The model under review builds one solid part; all positions refer to its coordinate system, in mm. Coordinates: 2 decimals unless noted, no trailing zeros. Loops run counter-clockwise (first coordinate to the right, second up) from the corner with the lowest first, then second, coordinate; pieces in that order, holes last. Notation, with made-up numbers: (-30.75, 23.5) - (26.25, 23.5) arc R18 ccw to (26.25, 42.5) - close; hole circle Ø5 at (58, 81.25). An arc over 180 degrees is marked (long way). Use a Markdown table: item, result. Add a question column.
1) Add section A-A, the plane z = -15.5. Give the boundary of the cut face in (x, y), and give its area (3 significant figures).
2) Clearance check with flat-ended pins moving along their axes: pin 1 (1 mm diameter, centred on x = -0.5, y = 0.5, fed in from -Z); pin 2 (2 mm diameter, centred on x = 0, y = 0, fed in from -Z); pin 3 (1 mm diameter, centred on x = -2, z = 10, fed in from -Y). State where each tip first meets the part, or that it passes through.
3) Add section C-C, the plane y = -1.95. Give the boundary of the cut face in (x, z), and give its area (3 significant figures).
4) Add section D-D, the plane x = 1.7. Give the boundary of the cut face in (y, z).
5) To check wall thickness, follow L1, parallel to Y at x = 0, z = -17; L2, parallel to Y at x = 0.5, z = -14; L3, parallel to Y at x = 1.6, z = -15. State the ranges of each line that lie inside material, in increasing order. Write a range as [from, to].
6) Add section B-B, the plane z = 6. Give the boundary of the cut face in (x, y).
```python
from build123d import *

# Parameters (mm, degrees)
SKETCH_6_R               = 2.5
EXTRUDE_2_DEPTH          = 19.3
M3X0_5_3_D               = 2.5
M3X0_5_3_DEPTH           = 8.5
M3X0_5_3_TIP             = 0.751075774
M3X0_5_3_ON_FACE_2_D     = 2.5
M3X0_5_3_ON_FACE_2_DEPTH = 8.5
M3X0_5_3_ON_FACE_2_TIP   = 0.751075774


with BuildPart() as part:
    # ｽｹｯﾁ6 → ﾎﾞｽ - 押し出し2 (new body, symmetric)
    with BuildSketch(Plane.XY):
        Circle(SKETCH_6_R)
    extrude(amount=EXTRUDE_2_DEPTH, both=True)

    # M3x0.5 ねじ穴3
    with Locations(Plane.XY.offset(19.3)):
        with Locations((0, 0)):
            Hole(M3X0_5_3_D / 2, depth=M3X0_5_3_DEPTH)
            with Locations((0, 0, -(M3X0_5_3_DEPTH + M3X0_5_3_TIP / 2))):  # 118° drill point
                Cone(0, M3X0_5_3_D / 2, M3X0_5_3_TIP, mode=Mode.SUBTRACT)

    # M3x0.5 ねじ穴3 on face 2
    with Locations(Plane(origin=(0, 0, -19.3), x_dir=(-1, 0, 0), z_dir=(0, 0, -1))):
        with Locations((0, 0)):
            Hole(M3X0_5_3_ON_FACE_2_D / 2, depth=M3X0_5_3_ON_FACE_2_DEPTH)
            with Locations((0, 0, -(M3X0_5_3_ON_FACE_2_DEPTH + M3X0_5_3_ON_FACE_2_TIP / 2))):  # 118° drill point
                Cone(0, M3X0_5_3_ON_FACE_2_D / 2, M3X0_5_3_ON_FACE_2_TIP, mode=Mode.SUBTRACT)


solid = part.part
```
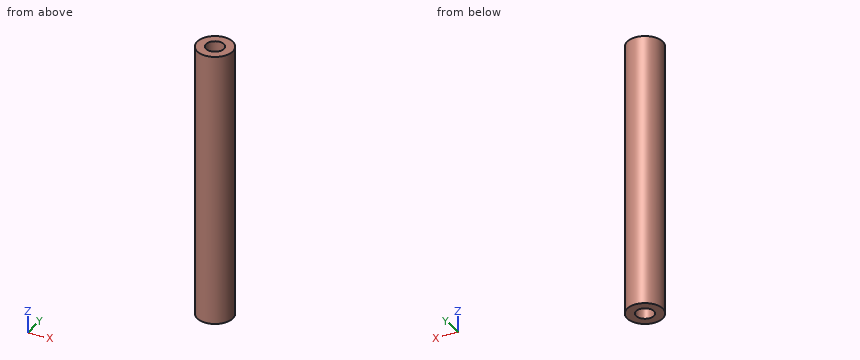
From the geometry:
| question | item | result |
|---|---|---|
| 1 | outline | circle Ø5 at (0, 0); hole circle Ø2.5 at (0, 0) |
| 1 | area | 14.7 mm^2 |
| 2 | pin 1 | stops at z = -10.77 |
| 2 | pin 2 | stops at z = -10.65 |
| 2 | pin 3 | stops at y = -2 |
| 3 | outline | (-1.56, -19.3) - (1.56, -19.3) - (1.56, 19.3) - (-1.56, 19.3) - close |
| 3 | area | 121 mm^2 |
| 4 | outline | (-1.83, -19.3) - (1.83, -19.3) - (1.83, 19.3) - (-1.83, 19.3) - close |
| 5 | L1 | y = [-2.5, -1.25], [1.25, 2.5] |
| 5 | L2 | y = [-2.45, -1.15], [1.15, 2.45] |
| 5 | L3 | y = [-1.92, 1.92] |
| 6 | outline | circle Ø5 at (0, 0) |
